The listing builds one solid part. Answer for the finished solid, in the listing's coordinates (mm). Give positions to 0.01 mm unless a question says otherwise; leave off trailing zeros. Order: outer loops, then holes, each group sorted by start corner. A loop starts at its lowest first (then second) coordinate and runs counter-clockwise, first axis right, second up. Notation, with made-up numbers: (-3.75, 56.25) - (4.25, 56.25) arc R30 ccw to (4.25, 78.25) - close; hole circle Ø3 at (53.5, -14.5). An arc over 180 degrees is marked (long way). Answer as a JSON object with one key per item and string values. Group by question number.
Q1. A cutting plane is placed at B-B, the plane x = 98.5. Give the vertices of the cut face in (y, z) (3 decimals), and give its area (3 significant figures).
Q2. A cutting plane is placed at A-A, the plane y = 2.1. Count the separate pieces of the cut face and the enclosed holes in it, and give its area (3 significant figures).
Q3. A cutting plane is placed at C-C, the plane z = -271.5. Give the vertices of the cut face in (x, y) (3 decimals).
Q4. Consider line 1 (Z direction, x = -11, y = 1.1); line 2 (X direction, y = 0.75, z = -622); line 3 (Z direction, x = 79, y = 1.8). Determine where each line is inside the solid, lowest interval first.
Q5. Given pin 1 (3 mm diameter, centred on x = -15.26, z = -634.68, fed in from -Y); pin 2 (1 mm diameter, centred on x = 37, y = 1, fed in from -Z), each flat-ended and moving along its own axis, determine where each tip first touches the part or whether it passes through.
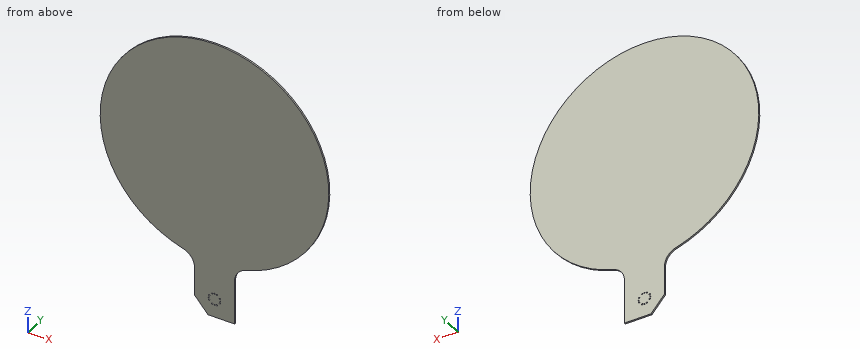
from build123d import *

# Parameters (mm, degrees)
BOSS_EXTRUDE1_DEPTH = 3.175
SKETCH20_R          = 1.25
SKETCH20_R_2        = 1
CUT_EXTRUDE1_DEPTH  = 4.175
CUT_EXTRUDE2_DEPTH  = 4.175


with BuildPart() as part:
    # Sketch1 → Boss-Extrude1 (new body)
    with BuildSketch(Plane(origin=(-1.297967049, 0, -318.957650502), x_dir=(1, 0, 0), z_dir=(0, 1, 0))):
        with BuildLine():
            Line((-41.969554108, 375.107652622), (34.230445892, 375.107652622))
            Line((34.230445892, 375.107652622), (34.230445892, 270.154369347))
            ThreePointArc((34.230445892, 270.154369347), (40.275943564, 252.093864975), (55.975900438, 241.312343077))
            ThreePointArc((55.975900438, 241.312343077), (-3.869554108, -185.292347378), (-63.715008653, 241.312343077))
            ThreePointArc((-63.715008653, 241.312343077), (-48.015051779, 252.093864975), (-41.969554108, 270.154369347))
            Line((-41.969554108, 270.154369347), (-41.969554108, 375.107652622))
        make_face()
    extrude(amount=BOSS_EXTRUDE1_DEPTH)

    # Sketch20 → Cut-Extrude1 (cut, through all)
    with BuildSketch(Plane(origin=(0, 3.175, 0), x_dir=(1, 0, 0), z_dir=(0, 1, 0))):
        with Locations((-15.257093255, 634.683461631)):
            Circle(SKETCH20_R)
        with Locations((-16.167521157, 639.065303124)):
            Circle(SKETCH20_R_2)
        with Locations((-15.257093255, 643.447144618)):
            Circle(SKETCH20_R)
        with Locations((-5.167521157, 628.065303124)):
            Circle(SKETCH20_R_2)
        with Locations((-9.549362651, 628.975731026)):
            Circle(SKETCH20_R)
        with Locations((-0.785679663, 628.975731026)):
            Circle(SKETCH20_R)
        with Locations((-9.549362651, 649.154875222)):
            Circle(SKETCH20_R)
        with Locations((-5.167521157, 650.065303124)):
            Circle(SKETCH20_R_2)
        with Locations((-0.785679663, 649.154875222)):
            Circle(SKETCH20_R)
        with Locations((4.922050941, 643.447144618)):
            Circle(SKETCH20_R)
        with Locations((5.832478843, 639.065303124)):
            Circle(SKETCH20_R_2)
        with Locations((4.922050941, 634.683461631)):
            Circle(SKETCH20_R)
    extrude(amount=-CUT_EXTRUDE1_DEPTH, mode=Mode.SUBTRACT)

    # Sketch21 → Cut-Extrude2 (cut, through all)
    with BuildSketch(Plane(origin=(0, 3.175, 0), x_dir=(1, 0, 0), z_dir=(0, 1, 0))):
        Polygon((32.932478843, 694.065303124), (-43.267521157, 694.065303124), (-43.267521157, 674.065303124), (-43.267521157, 644.143456202), (-17.515896333, 674.065303124), (32.932478843, 674.065303124), align=None)
    extrude(amount=-CUT_EXTRUDE2_DEPTH, mode=Mode.SUBTRACT)


solid = part.part
Reply:
{
 "1": {"outline": "(0, -542.37) - (3.175, -542.37) - (3.175, -159.96) - (0, -159.96) - close", "area": "1,210 mm^2"},
 "2": {"separate pieces": "1", "enclosed holes": "12", "area": "157,000 mm^2"},
 "3": {"outline": "(-207.553, 0) - (197.217, 0) - (197.217, 3.175) - (-207.553, 3.175) - close"},
 "4": {"line 1": "z = -674.07 to -133.74", "line 2": "x = -43.27 to 32.93", "line 3": "z = -551.72 to -150.61"},
 "5": {"pin 1": "stops at y = 0", "pin 2": "stops at z = -574.92"}
}
